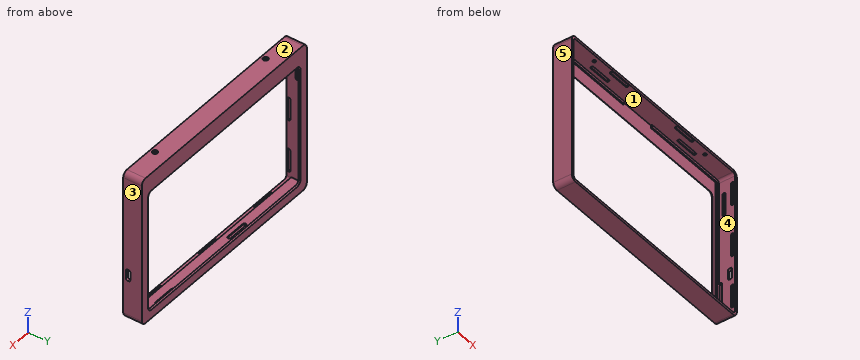
```python
from build123d import *

# Parameters (mm, degrees)
SKETCH_1_W           = 178.8
SKETCH_1_H           = 120.2
EXTRUDE_1_DEPTH      = 16
SHELL_1_T            = -2
SKETCH_4_W           = 178.821358432
SKETCH_4_H           = 120.2
CUT_EXTRUDE_2_DEPTH  = 1
SKETCH_2_W           = 163.4
SKETCH_2_H           = 96.92
CUT_EXTRUDE_1_DEPTH  = 1
FILLET_2_R           = 3
CHAMFER_1_SIZE       = 1
EXTRUDE_2_DEPTH      = 1
SKETCH1_W            = 178.8
SKETCH1_H            = 11
BOSS_EXTRUDE1_DEPTH  = 2.395
FILLET_1_R           = 4
CUT_EXTRUDE_3_DEPTH  = 1
CUT_EXTRUDE_4_DEPTH  = 1
CUT_EXTRUDE1_DEPTH   = 1
CUT_EXTRUDE_5_DEPTH  = 1
CUT_EXTRUDE_7_REACH  = 191.226
CUT_EXTRUDE_9_DEPTH  = 1
CUT_EXTRUDE3_DEPTH   = 1
CUT_EXTRUDE_10_DEPTH = 1
CUT_EXTRUDE2_DEPTH   = 1
FILLET1_R            = 2
SKETCH4_R            = 2
SKETCH4_R_2          = 1.25
CUT_EXTRUDE4_DEPTH   = 1
SKETCH4_3_R          = 1.25
CUT_EXTRUDE5_DEPTH   = 2
CUT_EXTRUDE6_DEPTH   = 1


with BuildPart() as part:
    # 草圖1 → 填料-伸長1 (new body)
    with BuildSketch(Plane(origin=(0, 0, 0), x_dir=(1, 0, 0), z_dir=(0, 1, 0))):
        Rectangle(SKETCH_1_W, SKETCH_1_H)
    extrude(amount=EXTRUDE_1_DEPTH)

    # 薄殼1
    shell_1_openings = [part.faces().sort_by_distance(p)[0] for p in [
        (0, 0, 0),
    ]]
    offset(amount=SHELL_1_T, openings=shell_1_openings, kind=Kind.INTERSECTION)

    # 草圖4 → 除料-伸長2 (cut)
    with BuildSketch(Plane(origin=(0, 16, 0), x_dir=(1, 0, 0), z_dir=(0, 1, 0))):
        Rectangle(SKETCH_4_W, SKETCH_4_H)
    extrude(amount=-CUT_EXTRUDE_2_DEPTH, mode=Mode.SUBTRACT)

    # 草圖2 → 除料-伸長1 (cut)
    with BuildSketch(Plane(origin=(0, 15, 0), x_dir=(1, 0, 0), z_dir=(0, 1, 0))):
        with Locations((0, 3.64)):
            Rectangle(SKETCH_2_W, SKETCH_2_H)
    extrude(amount=-CUT_EXTRUDE_1_DEPTH, mode=Mode.SUBTRACT)

    # 圓角2
    fillet_2_edges = [part.edges().sort_by_distance(p)[0] for p in [
        (81.7, 14.5, -52.1),
        (81.7, 14.5, 44.82),
        (-81.7, 14.5, 44.82),
        (-81.7, 14.5, -52.1),
    ]]
    fillet(fillet_2_edges, radius=FILLET_2_R)

    # 導角1
    chamfer_1_edges = [part.edges().sort_by_distance(p)[0] for p in [
        (0, 15, 44.82),
        (80.821320344, 15, 43.941320344),
        (-80.821320344, 15, 43.941320344),
        (81.7, 15, -3.64),
        (-81.7, 15, -3.64),
        (80.821320344, 15, -51.221320344),
        (-80.821320344, 15, -51.221320344),
        (0, 15, -52.1),
    ]]
    chamfer(chamfer_1_edges, length=CHAMFER_1_SIZE - 0.0001)  # a hair under: the kernel refuses the full size

    # 草圖13 → 填料-伸長2 (add)
    with BuildSketch(Plane.XZ.offset(-14)):
        Polygon((-87.4, 58.1), (-15, 58.1), (-15, 55.965), (-85.325, 55.965), (-85.325, -55.705), (85.325, -55.705), (85.325, 55.965), (15, 55.965), (15, 58.1), (87.4, 58.1), (87.4, -58.1), (-87.4, -58.1), align=None)
    extrude(amount=EXTRUDE_2_DEPTH)

    # Sketch1 → Boss-Extrude1 (add)
    with BuildSketch(Plane.XY.offset(-58.1)):
        with Locations((0, 9.5)):
            Rectangle(SKETCH1_W, SKETCH1_H)
    extrude(amount=BOSS_EXTRUDE1_DEPTH)

    # 圓角1
    fillet_1_edges = [part.edges().sort_by_distance(p)[0] for p in [
        (89.4, 7.5, 60.1),
        (-89.4, 7.5, 60.1),
        (-89.4, 7.5, -60.1),
        (89.4, 7.5, -60.1),
    ]]
    fillet(fillet_1_edges, radius=FILLET_1_R)

    # 草圖5 → 除料-伸長3 (cut)
    with BuildSketch(Plane.XY.offset(-55.705)):
        with BuildLine():
            Line((-30.1, 7.56), (-13.6, 7.56))
            ThreePointArc((-13.6, 7.56), (-12.35, 8.81), (-13.6, 10.06))
            Line((-13.6, 10.06), (-30.1, 10.06))
            ThreePointArc((-30.1, 10.06), (-31.35, 8.81), (-30.1, 7.56))
        make_face()
    extrude(amount=-CUT_EXTRUDE_3_DEPTH, mode=Mode.SUBTRACT)

    # 草圖6 → 除料-伸長4 (cut)
    with BuildSketch(Plane(origin=(-87.4, 0, 0), x_dir=(0, 0, -1), z_dir=(1, 0, 0))):
        with BuildLine():
            Line((-28.39, 10.06), (-44.89, 10.06))
            ThreePointArc((-44.89, 10.06), (-46.14, 8.81), (-44.89, 7.56))
            Line((-44.89, 7.56), (-28.39, 7.56))
            ThreePointArc((-28.39, 7.56), (-27.14, 8.81), (-28.39, 10.06))
        make_face()
    cut_extrude_4 = extrude(amount=-CUT_EXTRUDE_4_DEPTH, mode=Mode.SUBTRACT)

    # Mirror4: 除料-伸長4 across plane
    add(cut_extrude_4.mirror(Plane.ZY), mode=Mode.SUBTRACT)

    # 草圖6<4> → Cut-Extrude1 (cut)
    with BuildSketch(Plane(origin=(-87.4, 0, 0), x_dir=(0, 0, -1), z_dir=(1, 0, 0))):
        with BuildLine():
            ThreePointArc((44.89, 13), (46.14, 11.75), (44.89, 10.5))
            Line((44.89, 10.5), (28.39, 10.5))
            ThreePointArc((28.39, 10.5), (27.14, 11.75), (28.39, 13))
            Line((28.39, 13), (44.89, 13))
        make_face()
    cut_extrude1 = extrude(amount=-CUT_EXTRUDE1_DEPTH, mode=Mode.SUBTRACT)

    # Mirror2: Cut-Extrude1 across plane
    add(cut_extrude1.mirror(Plane.ZY), mode=Mode.SUBTRACT)

    # 草圖7 → 除料-伸長5 (cut)
    with BuildSketch(Plane(origin=(0, 0, 58.1), x_dir=(-1, 0, 0), z_dir=(0, 0, -1))):
        with BuildLine():
            Line((-55.28, 7.56), (-38.78, 7.56))
            ThreePointArc((-38.78, 7.56), (-37.53, 8.81), (-38.78, 10.06))
            Line((-38.78, 10.06), (-55.28, 10.06))
            ThreePointArc((-55.28, 10.06), (-56.53, 8.81), (-55.28, 7.56))
        make_face()
        with BuildLine():
            ThreePointArc((38.78, 7.56), (37.53, 8.81), (38.78, 10.06))
            Line((38.78, 10.06), (55.28, 10.06))
            ThreePointArc((55.28, 10.06), (56.53, 8.81), (55.28, 7.56))
            Line((55.28, 7.56), (38.78, 7.56))
        make_face()
    extrude(amount=-CUT_EXTRUDE_5_DEPTH, mode=Mode.SUBTRACT)

    # 草圖9 → 除料-伸長7 (cut, up to next)
    with BuildSketch(Plane(origin=(89.4, 0, 0), x_dir=(0, 0, -1), z_dir=(1, 0, 0)), mode=Mode.PRIVATE) as cut_extrude_7_sk1:
        with BuildLine():
            Line((26.59, 2.18), (19.79, 2.18))
            ThreePointArc((19.79, 2.18), (18.906116524, 2.546116524), (18.54, 3.43))
            Line((18.54, 3.43), (18.54, 4.43))
            ThreePointArc((18.54, 4.43), (18.906116524, 5.313883476), (19.79, 5.68))
            Line((19.79, 5.68), (26.59, 5.68))
            ThreePointArc((26.59, 5.68), (27.473883476, 5.313883476), (27.84, 4.43))
            Line((27.84, 4.43), (27.84, 3.43))
            ThreePointArc((27.84, 3.43), (27.473883476, 2.546116524), (26.59, 2.18))
        make_face()
    cut_extrude_7_tool1 = extrude(cut_extrude_7_sk1.sketch, amount=-CUT_EXTRUDE_7_REACH, mode=Mode.PRIVATE) & part.part
    add(cut_extrude_7_tool1.solids().sort_by_distance((89.4, 3.93, -23.19))[0], mode=Mode.SUBTRACT)

    # 草圖11 → 除料-伸長9 (cut)
    with BuildSketch(Plane.XY.offset(-58.1)):
        with BuildLine():
            Line((-8.25, 0.75), (8.25, 0.75))
            ThreePointArc((8.25, 0.75), (9.5, 2), (8.25, 3.25))
            Line((8.25, 3.25), (-8.25, 3.25))
            ThreePointArc((-8.25, 3.25), (-9.5, 2), (-8.25, 0.75))
        make_face()
    extrude(amount=-CUT_EXTRUDE_9_DEPTH, mode=Mode.SUBTRACT)

    # 草圖11<3> → Cut-Extrude3 (cut)
    with BuildSketch(Plane.XY.offset(-58.1)):
        with BuildLine():
            Line((51.75, 0.75), (68.25, 0.75))
            ThreePointArc((68.25, 0.75), (69.5, 2), (68.25, 3.25))
            Line((68.25, 3.25), (51.75, 3.25))
            ThreePointArc((51.75, 3.25), (50.5, 2), (51.75, 0.75))
        make_face()
        with BuildLine():
            Line((-68.25, 0.75), (-51.75, 0.75))
            ThreePointArc((-51.75, 0.75), (-50.5, 2), (-51.75, 3.25))
            Line((-51.75, 3.25), (-68.25, 3.25))
            ThreePointArc((-68.25, 3.25), (-69.5, 2), (-68.25, 0.75))
        make_face()
    extrude(amount=-CUT_EXTRUDE3_DEPTH, mode=Mode.SUBTRACT)

    # 草圖12 → 除料-伸長10 (cut)
    with BuildSketch(Plane(origin=(-87.4, 0, 0), x_dir=(0, 0, -1), z_dir=(1, 0, 0))):
        with BuildLine():
            Line((-8.25, 3.25), (8.25, 3.25))
            ThreePointArc((8.25, 3.25), (9.5, 2), (8.25, 0.75))
            Line((8.25, 0.75), (-8.25, 0.75))
            ThreePointArc((-8.25, 0.75), (-9.5, 2), (-8.25, 3.25))
        make_face()
        with BuildLine():
            Line((34.25, 3.25), (50.75, 3.25))
            ThreePointArc((50.75, 3.25), (52, 2), (50.75, 0.75))
            Line((50.75, 0.75), (34.25, 0.75))
            ThreePointArc((34.25, 0.75), (33, 2), (34.25, 3.25))
        make_face()
        with BuildLine():
            Line((-50.75, 3.25), (-34.25, 3.25))
            ThreePointArc((-34.25, 3.25), (-33, 2), (-34.25, 0.75))
            Line((-34.25, 0.75), (-50.75, 0.75))
            ThreePointArc((-50.75, 0.75), (-52, 2), (-50.75, 3.25))
        make_face()
    cut_extrude_10 = extrude(amount=-CUT_EXTRUDE_10_DEPTH, mode=Mode.SUBTRACT)

    # 鏡射2: 除料-伸長10 across plane
    add(cut_extrude_10.mirror(Plane.ZY), mode=Mode.SUBTRACT)

    # Sketch3 → Cut-Extrude2 (cut)
    with BuildSketch(Plane.XY.offset(-55.705)):
        with BuildLine():
            Line((51.900266162, 13), (68.400266162, 13))
            ThreePointArc((68.400266162, 13), (69.650266162, 11.75), (68.400266162, 10.5))
            Line((68.400266162, 10.5), (51.900266162, 10.5))
            ThreePointArc((51.900266162, 10.5), (50.650266162, 11.75), (51.900266162, 13))
        make_face()
    extrude(amount=-CUT_EXTRUDE2_DEPTH, mode=Mode.SUBTRACT)

    # Fillet1
    fillet1_edges = [part.edges().sort_by_distance(p)[0] for p in [
        (-87.4, 6.5, 58.1),
        (87.4, 6.5, 58.1),
        (-87.4, 2, -58.1),
        (87.4, 2, -58.1),
    ]]
    fillet(fillet1_edges, radius=FILLET1_R)

    # Sketch4 → Cut-Extrude4 (cut)
    # profile 1 of 2: a face of its own
    with BuildSketch(Plane.XY.offset(60.1)):
        with Locations((60, 3.75)):
            Circle(SKETCH4_R)
        with Locations((60, 3.75)):
            Circle(SKETCH4_R_2, mode=Mode.SUBTRACT)
    # profile 2 of 2: a face of its own
    with BuildSketch(Plane.XY.offset(60.1)):
        with Locations((60, 3.75)):
            Circle(SKETCH4_R_2)
    cut_extrude4 = extrude(amount=-CUT_EXTRUDE4_DEPTH, mode=Mode.SUBTRACT)

    # Sketch4<3> → Cut-Extrude5 (cut)
    with BuildSketch(Plane.XY.offset(60.1)):
        with Locations((60, 3.75)):
            Circle(SKETCH4_3_R)
    cut_extrude5 = extrude(amount=-CUT_EXTRUDE5_DEPTH, mode=Mode.SUBTRACT)

    # Mirror3: Cut-Extrude4, Cut-Extrude5 across plane
    add(cut_extrude4.mirror(Plane.ZY), mode=Mode.SUBTRACT)
    add(cut_extrude5.mirror(Plane.ZY), mode=Mode.SUBTRACT)

    # Sketch5 → Cut-Extrude6 (cut)
    with BuildSketch(Plane(origin=(0, 0, 58.1), x_dir=(-1, 0, 0), z_dir=(0, 0, -1))):
        with BuildLine():
            Line((27, 3.25), (43.5, 3.25))
            ThreePointArc((43.5, 3.25), (44.75, 2), (43.5, 0.75))
            Line((43.5, 0.75), (27, 0.75))
            ThreePointArc((27, 0.75), (25.75, 2), (27, 3.25))
        make_face()
        with BuildLine():
            Line((-27, 3.25), (-43.5, 3.25))
            ThreePointArc((-43.5, 3.25), (-44.75, 2), (-43.5, 0.75))
            Line((-43.5, 0.75), (-27, 0.75))
            ThreePointArc((-27, 0.75), (-25.75, 2), (-27, 3.25))
        make_face()
    extrude(amount=-CUT_EXTRUDE6_DEPTH, mode=Mode.SUBTRACT)


solid = part.part
```
Geometry check sheet. Reference: the model listing, model coordinates, mm. Face numbers are marked on the shaded views. A direction names the side the tool comes from. Coordinates: 2 decimals unless noted, no trailing zeros. One line per item, written item: value. Start each with the question number.
(1) Tool access check on the marked faces 4 and 5. Record the directions out of +Z, -Z, +X, -X, +Y, -Y that give a thin tool (end or side, any length) a straight path to the whole face; none if there is none.
(2) Scan lines: line 1 along Z through (x, y) = (-3.5, 5.5) (3 decimals); line 2 along X through (y, z) = (2.5, 14.5); line 3 along Z through (x, y) = (79, 1.5). Record each from-to range of solid material in increasing order. Write a range as [from, to].
(3) Release check for a two-part mould opening along X. For the marked faces 1, 2 and 3 record: released by +X, released by -X, zero draft, split by the parting line, or undercut.
Filled sheet:
1. face 4: -Y
1. face 5: +Z, -Z, -X, +Y, -Y
2. line 1: [-60.1, -55.705], [58.1, 60.1]
2. line 2: [-89.4, -87.4], [87.4, 89.4]
2. line 3: [-60.1, -58.1], [58.1, 60.1]
3. face 1: undercut
3. face 2: zero draft
3. face 3: released by +X
